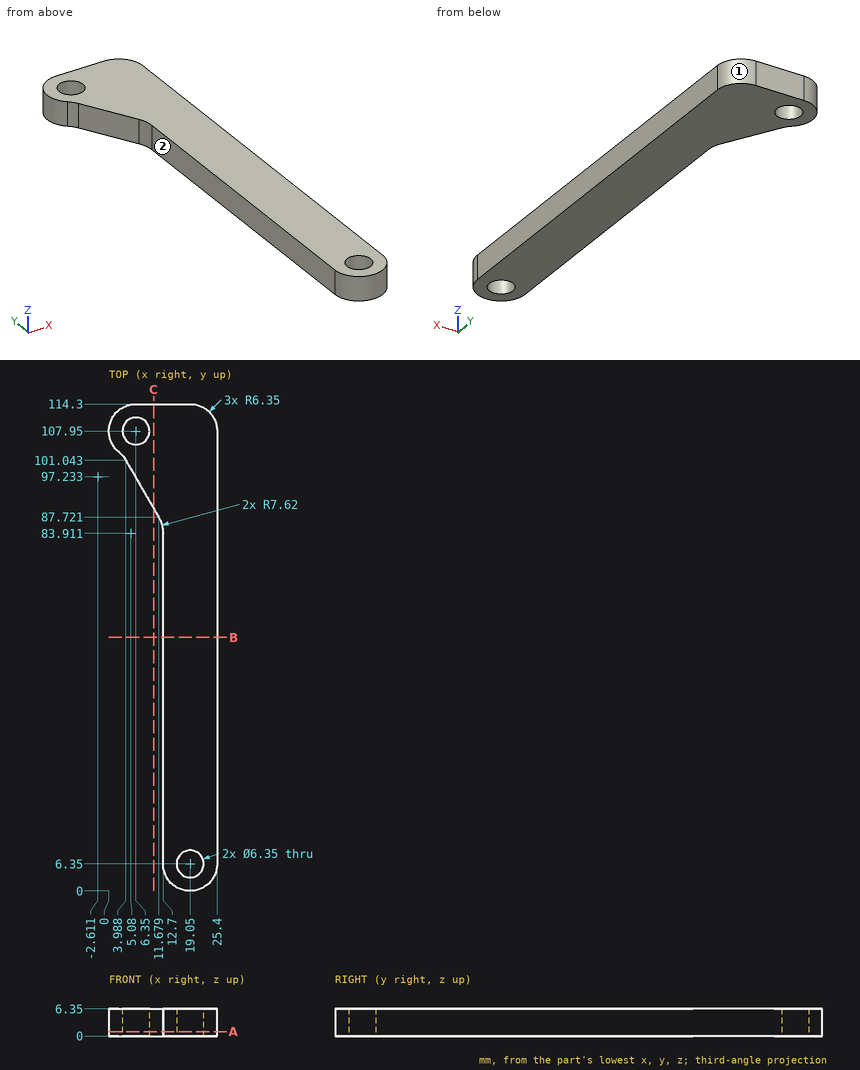
Could you check a few things on this drawing? It's one solid part, dimensions in mm from its lowest x, y, z. A direction names the side the tool comes from. Give positions to 0.01 mm unless a question says otherwise; leave off trailing zeros. Loops run counter-clockwise (first coordinate to the right, second up) from the corner with the lowest first, then second, coordinate; pieces in that order, holes last. Notation, with made-up numbers: M 61.5,-35 L 87.5,-35 A27 ccw 87.5,-13 Z; hole C 35,-18.5 d6. An arc over 180 degrees is marked long. One line per question, with ' | ' between items. Start each with the question number.
Q1. If we section it at A-A (z = 1): State how many separate pieces and enclosed holes the cut face has, plus the area to 3 significant figures.
Q2. If we section it at B-B (y = 59.5): Please give me the cut outline in (x, z).
Q3. For pin 1 Ø3 at (y, z) = (26, 3.5) entering from -X; pin 2 Ø3 at (x, z) = (8.5, 5.5) entering from -Y, each with a flat end and sliding along its axis, tell me the tip position at first contact or that it passes through.
Q4. For the marked faces 1 and 2, which set-ups out of +Z, -Z, +X, -X, +Y, -Y let a thin tool reach every point of the face, with its end or its side?
Q5. If I drill on line 1 (X direction, y = 107.95, z = 1.5) (1 decimal); line 2 (Y direction, x = 19.05, z = 4.25) (1 decimal); line 3 (X direction, y = 22, z = 6), over which ranges is the centre line in solid material (lowest first)? Write a range as from..to.
Q6. If we section it at C-C (x = 10.5): Please give me the cut outline in (y, z).
Computed:
1) separate pieces: 1 | enclosed holes: 2 | area: 1,580 mm²
2) outline: M 12.7,0 L 25.4,0 L 25.4,6.35 L 12.7,6.35 Z
3) pin 1: stops at x = 12.7 | pin 2: stops at y = 90.63
4) face 1: +Z, -Z, +X, +Y | face 2: +Z, -Z, -X, -Y
5) line 1: x = 0..3.2, 9.5..25.4 | line 2: y = 0..3.2, 9.5..114.3 | line 3: x = 12.7..25.4
6) outline: M 89.76,0 L 114.3,0 L 114.3,6.35 L 89.76,6.35 Z
